Work out the finished part from the listing and answer in its coordinate system (mm). Give positions to 0.01 mm unless a question says otherwise; leave off trailing zeros. Loops run counter-clockwise (first coordinate to the right, second up) from the corner with the lowest first, then second, coordinate; pieces in that order, holes last.
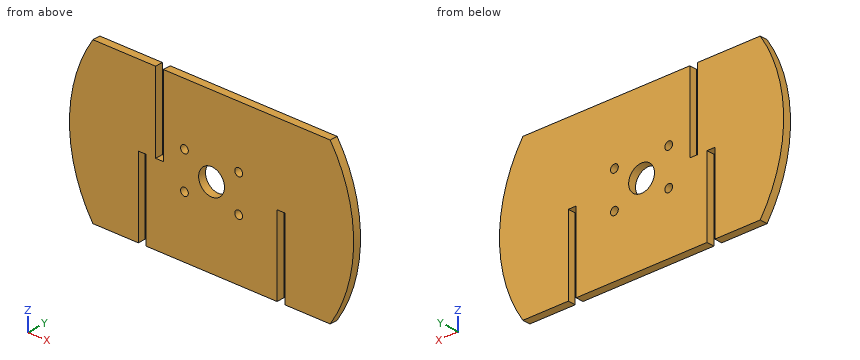
from build123d import *

# Parameters (mm, degrees)
BOSS_EXTRUDE1_DEPTH = 3
SKETCH4_R           = 5
CUT_EXTRUDE1_DEPTH  = 3
SKETCH6_R           = 1.5
CUT_EXTRUDE2_DEPTH  = 3
CUT_EXTRUDE3_DEPTH  = 3
SKETCH8_W           = 3
SKETCH8_H           = 30.3
CUT_EXTRUDE4_DEPTH  = 3


with BuildPart() as part:
    # Sketch3 → Boss-Extrude1 (new body)
    with BuildSketch(Plane(origin=(0, 0, 0), x_dir=(1, 0, 0), z_dir=(0, 1, 0))):
        with BuildLine():
            Line((-42.11236018, 3.702994226), (-22.11236018, 3.702994226))
            Line((-22.11236018, 3.702994226), (-22.11236018, -26.497005774))
            Line((-22.11236018, -26.497005774), (-19.11236018, -26.497005774))
            Line((-19.11236018, -26.497005774), (-19.11236018, 3.702994226))
            Line((-19.11236018, 3.702994226), (-15.45236018, 3.702994226))
            Line((-15.45236018, 3.702994226), (-12.45236018, 3.702994226))
            Line((-12.45236018, 3.702994226), (31.57763982, 3.702994226))
            Line((31.57763982, 3.702994226), (31.57763982, -26.497005774))
            Line((31.57763982, -26.497005774), (34.57763982, -26.497005774))
            Line((34.57763982, -26.497005774), (34.57763982, 3.702994226))
            Line((34.57763982, 3.702994226), (54.57763982, 3.702994226))
            ThreePointArc((54.57763982, 3.702994226), (61.648707631, 0.774062038), (64.57763982, -6.297005774))
            Line((64.57763982, -6.297005774), (64.57763982, -46.797005774))
            ThreePointArc((64.57763982, -46.797005774), (61.648707631, -53.868073586), (54.57763982, -56.797005774))
            Line((54.57763982, -56.797005774), (-42.11236018, -56.797005774))
            ThreePointArc((-42.11236018, -56.797005774), (-49.183427992, -53.868073586), (-52.11236018, -46.797005774))
            Line((-52.11236018, -46.797005774), (-52.11236018, -6.297005774))
            ThreePointArc((-52.11236018, -6.297005774), (-49.183427992, 0.774062038), (-42.11236018, 3.702994226))
        make_face()
    extrude(amount=BOSS_EXTRUDE1_DEPTH)

    # Sketch4 → Cut-Extrude1 (cut)
    with BuildSketch(Plane(origin=(0, 3, 0), x_dir=(1, 0, 0), z_dir=(0, 1, 0))):
        with Locations(Location((6.23263982, -26.547005774, 0), (0, 0, 270))):
            Circle(SKETCH4_R)
    extrude(amount=-CUT_EXTRUDE1_DEPTH, mode=Mode.SUBTRACT)

    # Sketch6 → Cut-Extrude2 (cut)
    with BuildSketch(Plane(origin=(0, 3, 0), x_dir=(1, 0, 0), z_dir=(0, 1, 0))):
        with Locations(Location((-4.26736018, -19.497005774, 0), (0, 0, 270))):
            Circle(SKETCH6_R)
        with Locations(Location((-4.26736018, -33.497005774, 0), (0, 0, 270))):
            Circle(SKETCH6_R)
        with Locations(Location((16.73263982, -19.497005774, 0), (0, 0, 270))):
            Circle(SKETCH6_R)
        with Locations(Location((16.73263982, -33.497005774, 0), (0, 0, 270))):
            Circle(SKETCH6_R)
    extrude(amount=-CUT_EXTRUDE2_DEPTH, mode=Mode.SUBTRACT)

    # Sketch7 → Cut-Extrude3 (cut)
    with BuildSketch(Plane(origin=(0, 3, 0), x_dir=(1, 0, 0), z_dir=(0, 1, 0))):
        with BuildLine():
            Line((52.166695813, 3.702994226), (73.459164028, 3.702994226))
            Line((73.459164028, 3.702994226), (73.459164028, -56.797005774))
            Line((73.459164028, -56.797005774), (52.166695813, -56.797005774))
            ThreePointArc((52.166695813, -56.797005774), (61.23263982, -26.547005774), (52.166695813, 3.702994226))
        make_face()
        with BuildLine():
            Line((-39.701416174, 3.702994226), (-60.819947715, 3.702994226))
            Line((-60.819947715, 3.702994226), (-60.819947715, -56.797005774))
            Line((-60.819947715, -56.797005774), (-39.701416174, -56.797005774))
            ThreePointArc((-39.701416174, -56.797005774), (-48.76736018, -26.547005774), (-39.701416174, 3.702994226))
        make_face()
    extrude(amount=-CUT_EXTRUDE3_DEPTH, mode=Mode.SUBTRACT)

    # Sketch8 → Cut-Extrude4 (cut)
    with BuildSketch(Plane(origin=(0, 3, 0), x_dir=(1, 0, 0), z_dir=(0, 1, 0))):
        with Locations((-13.95236018, -41.647005774)):
            Rectangle(SKETCH8_W, SKETCH8_H)
    extrude(amount=-CUT_EXTRUDE4_DEPTH, mode=Mode.SUBTRACT)


solid = part.part
Item 1: Find section A-A, the plane z = 30. Write down the section's boundary in (x, y), plus the area to 3 significant figures.
Item 2: Find section D-D, the plane y = 2.15. Write down the section's boundary in (x, z), plus the area to 3 significant figures.
Item 3: Flat-ended cylindrical pins translate along their axes: pin 1 Ø1.5 at (y, z) = (1.5, 40.5) entering from +X; pin 2 Ø0.9 at (y, z) = (1, 43.5) entering from -X; pin 3 Ø0.9 at (x, y) = (-14.5, 1) entering from +Z. Find the tip coordinate at first contact, or state that the pin passes through.
Item 4: Find section B-B, the plane x = 5. Write down the section's boundary in (y, z).
Item 5: Find section C-C, the plane z = 48.5. Write down the section's boundary in (x, y).
Item 6: Consider line 1 (X direction, y = 0.8, z = 27); line 2 (X direction, y = 2.55, z = 31); line 3 (Z direction, x = 32, y = 2.3). Determine where each line is inside the solid, lowest interval first.
Ans:
1. outline: (-48.66, 0) - (-15.45, 0) - (-15.45, 3) - (-48.66, 3) - close; (-12.45, 0) - (2.62, 0) - (2.62, 3) - (-12.45, 3) - close; (9.85, 0) - (61.12, 0) - (61.12, 3) - (9.85, 3) - close
1. area: 299 mm2
2. outline: (-39.7, -3.7) - (-22.11, -3.7) - (-22.11, 26.5) - (-19.11, 26.5) - (-19.11, -3.7) - (31.58, -3.7) - (31.58, 26.5) - (34.58, 26.5) - (34.58, -3.7) - (52.17, -3.7) arc R55 ccw to (52.17, 56.8) - (-12.45, 56.8) - (-12.45, 26.5) - (-15.45, 26.5) - (-15.45, 56.8) - (-39.7, 56.8) arc R55 ccw to start; hole circle Ø3 at (-4.27, 19.5); hole circle Ø3 at (-4.27, 33.5); hole circle Ø10 at (6.23, 26.55); hole circle Ø3 at (16.73, 19.5); hole circle Ø3 at (16.73, 33.5)
2. area: 5,920 mm2
3. pin 1: stops at x = 59.62
3. pin 2: stops at x = -46.23
3. pin 3: stops at z = 26.5
4. outline: (0, -3.7) - (3, -3.7) - (3, 21.7) - (0, 21.7) - close; (0, 31.39) - (3, 31.39) - (3, 56.8) - (0, 56.8) - close
5. outline: (-44.2, 0) - (-15.45, 0) - (-15.45, 3) - (-44.2, 3) - close; (-12.45, 0) - (56.66, 0) - (56.66, 3) - (-12.45, 3) - close
6. line 1: x = -48.77 to -15.45, -12.45 to 1.25, 11.21 to 61.23
6. line 2: x = -48.59 to -15.45, -12.45 to 3.96, 8.51 to 61.05
6. line 3: z = 26.5 to 56.8
